Autodesk Inventor part; units mm, degrees
ref_plane "YZ Plane" through (0, 0, 0) normal (1, 0, 0) x (0, 1, 0)
ref_plane "XZ Plane" through (0, 0, 0) normal (0, 1, 0) x (-1, 0, 0)
ref_plane "XY Plane" through (0, 0, 0) normal (0, 0, 1) x (1, 0, 0)
sketch "スケッチ1" plane through (0, 0, 0) normal (0, 1, 0) x (-1, 0, 0)
  line L0 (0, 0) -> (140, 0)
  line L1 (140, -65) -> (0, -65)
  line L2 (0, -65) -> (0, 0)
  line L3 (124.5, 0) -> (118.5, 0)
  line L4 (118.5, 0) -> (118.5, -6)
  line L5 (118.5, -6) -> (124.5, -6)
  line L6 (124.5, -6) -> (124.5, 0)
  line L7 (124.5, -65) -> (118.5, -65)
  line L8 (118.5, -65) -> (118.5, -59)
  line L9 (118.5, -59) -> (124.5, -59)
  line L10 (124.5, -59) -> (124.5, -65)
  line L11 (0, -45) -> (25, -65)
  line L12 (0, -20) -> (25, 0)
  line L13 (60, -25) -> (55, -25)
  line L14 (55, -25) -> (55, -40)
  line L15 (55, -40) -> (60, -40)
  line L16 (60, -40) -> (60, -25)
  line L17 (140, -70) -> (161, -70)
  line L18 (161, -70) -> (161, 5)
  line L19 (161, 5) -> (140, 5)
  line L20 (140, -65) -> (140, -70)
  line L21 (140, 0) -> (140, 5)
  point P0 (124.5, -3)
  point P1 (124.5, -62)
  point P2 (118.5, 0)
  dimension "d0" = 140
  dimension "d1" = 65
  dimension "d61" = 6
  dimension "d62" = 6
  dimension "d63" = 6
  dimension "d64" = 6
  dimension "d66" = 20
  dimension "d67" = 20
  dimension "d68" = 25
  dimension "d70" = 5
  dimension "d71" = 15
  dimension "d73" = 25
  dimension "d103" = 21
  dimension "d104" = 75
  dimension "d105" = 5
extrude "押し出し1" add sketch "スケッチ1" along normal blind 3 contours L0 L4 L5 L6 L21 L19 L18 L17 L20 L1 L10 L9 L8 L11 L2 L12
sketch "スケッチ2" plane through (0, 3, 0) normal (0, 1, 0) x (1, 0, 0)
  line L0 (-140, 0) -> (0, 0)
  line L1 (-25, 65) -> (-140, 65)
  line L2 (-140, 65) -> (-140, 70)
  point P0 (-121.5, 12.5)
  point P1 (0, 65)
  point P2 (-121.5, 52.5)
  dimension "d9" = 12.5
  dimension "d55" = 12.5
  dimension "d69" = 40
  dimension "d107" = 18.5
hole "穴1" at (-121.5, 3, -12.5) at (-121.5, 3, -52.5) direction (0, -1, 0) diameter 3.2 end through all
sketch "スケッチ3" plane through (0, 3, 0) normal (0, 1, 0) x (1, 0, 0)
  line L0 (-140, 0) -> (0, 0)
  line L1 (-25, 65) -> (-140, 65)
  line L2 (0, 0) -> (0, 45)
  point P0 (-35, 22.5)
  point P1 (-35, 42.5)
  point P2 (-15, 42.5)
  point P3 (-15, 22.5)
  point P4 (0, 65)
  dimension "d20" = 20
  dimension "d21" = 20
  dimension "d22" = 22.5
  dimension "d24" = 15
hole "穴2" at (-35, 3, -22.5) at (-35, 3, -42.5) at (-15, 3, -42.5) at (-15, 3, -22.5) direction (0, -1, 0) diameter 3.2 end through all
sketch "スケッチ4" plane through (0, 3, 0) normal (0, 1, 0) x (1, 0, 0)
  line L0 (-25, 65) -> (-140, 65)
  line L1 (0, 0) -> (0, 45)
  point P0 (-5, 42.5)
  point P1 (-5, 32.5)
  point P2 (-5, 22.5)
  point P3 (0, 65)
  dimension "d32" = 10
  dimension "d33" = 10
  dimension "d34" = 32.5
  dimension "d35" = 5
hole "穴3" at (-5, 3, -42.5) at (-5, 3, -32.5) at (-5, 3, -22.5) direction (0, -1, 0) diameter 3.2 end through all
sketch "スケッチ5" plane through (0, 3, 0) normal (0, 1, 0) x (1, 0, 0)
  line L0 (-25, 65) -> (-140, 65)
  line L1 (-140, 65) -> (-140, 0)
  line L2 (-140, 65) -> (-140, 70)
  point P0 (0, 0)
  point P1 (-94, 53)
  point P2 (-28, 53)
  point P3 (-28, 12)
  point P4 (-94, 12)
  point P5 (0, 65)
  dimension "d43" = 66
  dimension "d44" = 41
  dimension "d46" = 12
  dimension "d106" = 46
hole "穴4" at (-94, 3, -53) at (-28, 3, -53) at (-28, 3, -12) at (-94, 3, -12) direction (0, -1, 0) diameter 3.2 end through all
sketch "スケッチ8" plane through (0, 3, 0) normal (0, 1, 0) x (1, 0, 0)
  line L0 (-140, 70) -> (-161, 70)
  line L1 (-161, 70) -> (-161, -5)
  point P0 (0, 0)
  point P1 (-150.5, 59.35)
  point P2 (-150.5, 5.65)
  dimension "d108" = 10.65
  dimension "d109" = 10.5
  dimension "d110" = 53.7
hole "穴5" at (-150.5, 3, -59.35) at (-150.5, 3, -5.65) direction (0, -1, 0) diameter 3.2 end through all
sketch "スケッチ7" plane through (0, 3, 0) normal (0, 1, 0) x (1, 0, 0)
  line L0 (-140, 65) -> (-124.5, 65)
  line L1 (-124.5, 59) -> (-124.5, 65)
  line L2 (-124.5, 65) -> (-124.5, 59)
  line L3 (-118.5, 59) -> (-124.5, 59)
  line L4 (-124.5, 59) -> (-118.5, 59)
  line L5 (-118.5, 65) -> (-118.5, 59)
  line L6 (-118.5, 59) -> (-118.5, 65)
  line L7 (-118.5, 65) -> (-60.0781, 65)
  line L8 (0, 39.7809) -> (0, 25.2191)
  line L9 (-60.0781, 0) -> (-118.5, 0)
  line L10 (-118.5, 0) -> (-118.5, 6)
  line L11 (-118.5, 6) -> (-124.5, 6)
  line L12 (-124.5, 6) -> (-124.5, 0)
  line L13 (-124.5, 0) -> (-140, 0)
  circle A0 centre (-121.5, 52.5) radius 1.6
  circle A1 centre (-121.5, 12.5) radius 1.6
  line L14 (-60, 40) -> (-55, 40)
  line L15 (-55, 40) -> (-55, 25)
  line L16 (-60, 40) -> (-55, 40)
  line L17 (-55, 40) -> (-55, 25)
  line L18 (-55, 25) -> (-60, 25)
  line L19 (-60, 25) -> (-60, 40)
  circle A2 centre (-94, 53) radius 1.6
  circle A3 centre (-94, 12) radius 1.6
  circle A4 centre (-28, 53) radius 1.6
  circle A5 centre (-28, 12) radius 1.6
  circle A6 centre (-35, 42.5) radius 1.6
  circle A7 centre (-15, 42.5) radius 1.6
  circle A8 centre (-35, 22.5) radius 1.6
  circle A9 centre (-15, 22.5) radius 1.6
  circle A10 centre (-5, 42.5) radius 1.6
  circle A11 centre (-5, 32.5) radius 1.6
  circle A12 centre (-5, 22.5) radius 1.6
  line L20 (-140, 65) -> (-140, 70)
  line L21 (-140, 70) -> (-161, 70)
  line L22 (-140, 70) -> (-161, 70)
  line L23 (-161, 70) -> (-161, -5)
  line L24 (-161, 70) -> (-161, -5)
  line L25 (-161, -5) -> (-140, -5)
  line L26 (-161, -5) -> (-140, -5)
  line L27 (-140, -5) -> (-140, 0)
  line L28 (-140, -5) -> (-140, 0)
  circle A13 centre (-150.5, 59.35) radius 1.6
  circle A14 centre (-150.5, 59.35) radius 1.6
  circle A15 centre (-150.5, 5.65) radius 1.6
  arc A16 (-60.0781, 0) -> (-4.4358, 16.9101) centre (-60.0781, 100) ccw
  arc A17 (-4.4358, 48.0899) -> (-60.0781, 65) centre (-60.0781, -35) ccw
  arc A18 (0, 39.7809) -> (-4.4358, 48.0899) centre (-10, 39.7809) ccw
  arc A19 (-4.4358, 16.9101) -> (0, 25.2191) centre (-10, 25.2191) ccw
  point P0 (0, 0)
  point P1 (-25, 65)
  point P2 (0, 45)
  point P3 (-25, 0)
  point P4 (0, 20)
  dimension "d74" = 3.2
  dimension "d75" = 3.2
  dimension "d77" = 40
  dimension "d79" = 3.2
  dimension "d80" = 3.2
  dimension "d81" = 3.2
  dimension "d82" = 3.2
  dimension "d83" = 41
  dimension "d86" = 66
  dimension "d87" = 3.2
  dimension "d88" = 3.2
  dimension "d89" = 3.2
  dimension "d90" = 3.2
  dimension "d91" = 20
  dimension "d92" = 20
  dimension "d94" = 15
  dimension "d95" = 3.2
  dimension "d96" = 3.2
  dimension "d97" = 3.2
  dimension "d98" = 10
  dimension "d99" = 10
  dimension "d100" = 5
  dimension "d118" = 18.5
  dimension "d119" = 46
  dimension "d121" = 161
  dimension "d123" = 3.2
  dimension "d124" = 3.2
  dimension "d125" = 10.5
  dimension "d126" = 10.65
  dimension "d127" = 53.7
  dimension "d129" = 6
  dimension "d133" = 100
  dimension "d134" = 10
  dimension "d138" = 32.5
  dimension "d139" = 22.5
  dimension "d140" = 12
  dimension "d141" = 16.9101
  dimension "d142" = 16.9101
fillet "フィレット1" radius 100 1 edges at (-25, 1.5, 0)
fillet "フィレット2" radius 100 1 edges at (-25, 1.5, -65)
fillet "フィレット3" radius 10 1 edges at (0, 1.5, -20)
fillet "フィレット4" radius 10 1 edges at (0, 1.5, -45)
properties material "アクリル"
Geometry check sheet. Reference: the model listing, model coordinates, mm. A direction names the side the tool comes from. Coordinates: 2 decimals unless noted, no trailing zeros. Order: outer loops, then holes, each group sorted by start corner. A loop starts at its lowest first (then second) coordinate and runs counter-clockwise, first axis right, second up. Notation, with made-up numbers: (-32.75, -16.75) -> (-22.75, -16.75) arc R16 cw to (-22.75, 6.25) -> close; hole circle Ø9 at (77.25, -28). An arc over 180 degrees is marked (long way). Use a Markdown table: item, result. Add a question column.
1. Mould release check, pull along X, two halves, no side actions. Record for faces 5 (the face through (-33.58, 1.48, -41.76)), 6 (the face through (-132, 1, 0)), 7 (the face through (-140, 1, -67)): pulls with the +X half, pulls with the -X half, needs draft (parallel to the pull), parting line crosses it, or undercut.
2. Set-up check for faces 1 (the face through (-90, 1, -65)), 2 (the face through (0, 1, -33)), 3 (the face through (-124.5, 1, -62)), 4 (the face through (-58, 1, -25)): record each of +Z, -Z, +X, -X, +Y, -Y from which the full face is reachable in a straight line by a thin tool's end or side.
3. Material ranges on L1, parallel to Z at x = -121.5, y = 1.15; L2, parallel to Z at x = -150.5, y = 1.05; L3, parallel to X at y = 0.65, z = -43.5, recorded low to high.
4. Cross-section at A-A (x = -150.5). Enter the section's corners in (y, z), and give its area (3 significant figures).
5. Cross-section at C-C (z = -2). Enter the section's corners in (x, y).
6. Cross-section at D-D (y = 1.9). Give the number of separate pieces and of enclosed holes in the cut face, and give its area (3 significant figures).
7. Cross-section at B-B (z = -32.5). Enter the section's corners in (x, y), and give its area (3 significant figures).
8. Go/stop test with flat-tipped pins: pin 1 Ø1.5 at (x, y) = (-135, 1.5) entering from -Z; pin 2 Ø1.5 at (x, y) = (-51.5, 2) entering from -Z; pin 3 Ø1.5 at (x, y) = (-78.5, 0.5) entering from +Z. Record where each tip stops, or that it passes through.
Filled sheet:
| question | item | result |
|---|---|---|
| 1 | face 5 | undercut |
| 1 | face 6 | needs draft |
| 1 | face 7 | pulls with the +X half |
| 2 | face 1 | -Z, +X, +Y, -Y |
| 2 | face 2 | +Z, -Z, +X, +Y, -Y |
| 2 | face 3 | -Z, +Y, -Y |
| 2 | face 4 | +Y, -Y |
| 3 | L1 | -59 to -54.1, -50.9 to -14.1, -10.9 to -6 |
| 3 | L2 | -70 to -60.95, -57.75 to -7.25, -4.05 to 5 |
| 3 | L3 | -161 to -36.25, -33.75 to -16.25, -13.75 to -6.25, -3.75 to -0.7 |
| 4 | outline | (0, -70) -> (3, -70) -> (3, -60.95) -> (0, -60.95) -> close; (0, -57.75) -> (3, -57.75) -> (3, -7.25) -> (0, -7.25) -> close; (0, -4.05) -> (3, -4.05) -> (3, 5) -> (0, 5) -> close |
| 4 | area | 206 mm2 |
| 5 | outline | (-161, 0) -> (-124.5, 0) -> (-124.5, 3) -> (-161, 3) -> close; (-118.5, 0) -> (-40.1, 0) -> (-40.1, 3) -> (-118.5, 3) -> close |
| 6 | separate pieces | 1 |
| 6 | enclosed holes | 16 |
| 6 | area | 9,630 mm2 |
| 7 | outline | (-161, 0) -> (-60, 0) -> (-60, 3) -> (-161, 3) -> close; (-55, 0) -> (-6.6, 0) -> (-6.6, 3) -> (-55, 3) -> close; (-3.4, 0) -> (0, 0) -> (0, 3) -> (-3.4, 3) -> close |
| 7 | area | 458 mm2 |
| 8 | pin 1 | z = -65 |
| 8 | pin 2 | z = -64.7 |
| 8 | pin 3 | z = 0 |
